Answer from the drawing. Dimensions are ordinates in mm from the lowest x, y and z of the part. Round coordinates to 2 decimals unless told otherwise and drop trailing zeros. Write each loop counter-clockwise with the first axis right and the second up, starting at its lowest first coordinate (ties: lowest second). Pieces come first, ordered by that corner, then holes. Notation, with made-up numbers: (51, 2.25) - (108, 2.25) arc R17 cw to (108, 33.25) - close; hole circle Ø7 at (-15.75, -10). An arc over 180 degrees is marked (long way). One line per item, written item: value. Start each with the question number.
(1) Flat-ended cylindrical pins translate along their axes: pin 1 Ø1 at (y, z) = (1, 74) entering from +X (3 decimals); pin 2 Ø12 at (x, z) = (40.5, 79) entering from -Y; pin 3 Ø1.6 at (y, z) = (2, 95.5) entering from -X (3 decimals). Find the tip coordinate at first contact, or state that the pin passes through.
(2) Find the intervals of material crossed by L1, parallel to Z at x = 43.5, y = 2.85; L2, parallel to Z at x = 19.5, y = 1.75 (3 decimals); L3, parallel to X at y = 1.25, z = 30 (3 decimals), in increasing order.
(3) A cutting plane is placed at A-A, the plane x = 11.5. Determine the outline of the cut face in (y, z) (3 decimals), plus the area to 3 significant figures.
(4) A cutting plane is placed at B-B, the plane z = 30. Determine the outline of the cut face in (x, y) (3 decimals), plus the area to 3 significant figures.
(5) A cutting plane is placed at C-C, the plane y = 0.7. State how many separate pieces and enclosed holes the cut face has, plus the area to 3 significant figures.
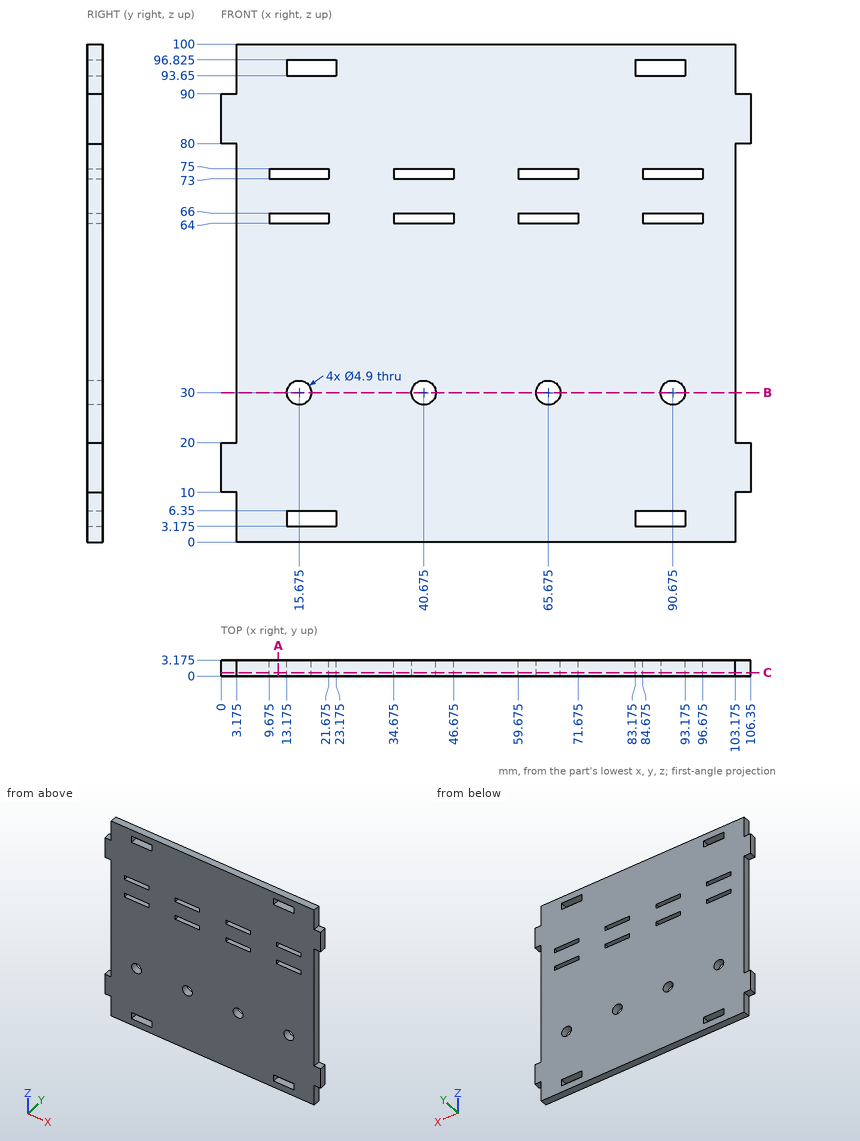
Here are the results:
1. pin 1: x = 103.175
1. pin 2: y = 0
1. pin 3: x = 3.175
2. L1: 0 to 64, 66 to 73, 75 to 100
2. L2: 0 to 3.175, 6.35 to 64, 66 to 73, 75 to 93.65, 96.825 to 100
2. L3: 3.175 to 13.225, 18.125 to 38.225, 43.125 to 63.225, 68.125 to 88.225, 93.125 to 103.175
3. outline: (0, 0) - (3.175, 0) - (3.175, 64) - (0, 64) - close; (0, 66) - (3.175, 66) - (3.175, 73) - (0, 73) - close; (0, 75) - (3.175, 75) - (3.175, 100) - (0, 100) - close
3. area: 305 mm²
4. outline: (3.175, 0) - (13.225, 0) - (13.225, 3.175) - (3.175, 3.175) - close; (18.125, 0) - (38.225, 0) - (38.225, 3.175) - (18.125, 3.175) - close; (43.125, 0) - (63.225, 0) - (63.225, 3.175) - (43.125, 3.175) - close; (68.125, 0) - (88.225, 0) - (88.225, 3.175) - (68.125, 3.175) - close; (93.125, 0) - (103.175, 0) - (103.175, 3.175) - (93.125, 3.175) - close
4. area: 255 mm²
5. separate pieces: 1
5. enclosed holes: 16
5. area: 9,730 mm²
